Input: dimensioned drawing with shaded views. Units: mm. Origin: part minimum x, y, z. Give positions to 0.01 mm unless a question says otherwise; leave off trailing zeros. Order: outer loops, then holes, each group sorted by start corner. A loop starts at its lowest first (then second) coordinate and runs counter-clockwise, first axis right, second up. Notation, with made-up numbers: (-16, -26) -> (39, -26) arc R13 ccw to (39, -14) -> close; hole circle Ø10 at (70.25, -14). An arc over 180 degrees is marked (long way). One line per question, with ' | ' between items. Start each with the question number.
(1) Ray query, L1, parallel to X at y = 5.75, z = 3.45; L2, parallel to Y at x = 4.25, z = 1.85 (1 decimal); L3, parallel to Y at x = 5.5, z = 4.85 (1 decimal). Return the intervals inside material, ascending.
(2) First-contact query: pin 1 Ø1.5 at (x, z) = (1.5, 1) entering from -Y; pin 2 Ø2 at (x, z) = (8, 1) entering from +Y; pin 3 Ø2 at (x, z) = (9, 4) entering from +Y (1 decimal). Flat tips, straight axial feed; report the tip coordinate or a pass-through.
(3) Section A-A (z = 4.4). Return loops of the section in (x, y).
(4) Mould query, pull axis Y, two halves, no side actions, for the marked faces 1, 2 and 3. Classes: +Y half, -Y half, draft (parallel to the pull), parting line (faces both ways), or undercut.
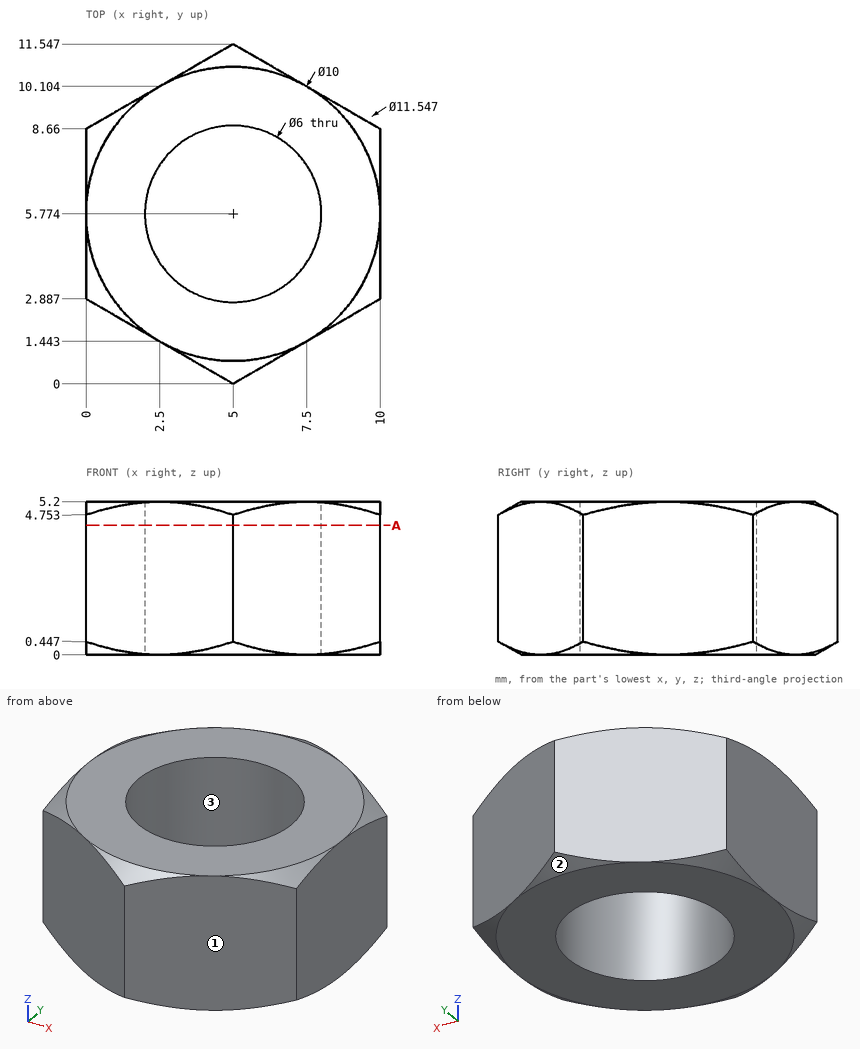
Response:
1) L1: x = 0 to 2, 8 to 10 | L2: y = 0.4 to 2.9, 8.7 to 11.1 | L3: y = 0.3 to 2.8, 8.7 to 11.3
2) pin 1: stops at y = 1.59 | pin 2: stops at y = 10.39 | pin 3: stops at y = 9.8
3) outline: (0, 2.89) -> (5, 0) -> (10, 2.89) -> (10, 8.66) -> (5, 11.55) -> (0, 8.66) -> close; hole circle Ø6 at (5, 5.77)
4) face 1: -Y half | face 2: +Y half | face 3: undercut
